from build123d import *

# Parameters (mm, degrees)
BOSS_EXTRUDE1_START            = -131.7625
BOSS_EXTRUDE1_DEPTH            = 60.325
F_5_0MM_DOWEL_HOLE1_AT_2_COUNT = 2
F_5_0MM_DOWEL_HOLE1_AT_2_PITCH = 12.7
F_5_0MM_DOWEL_HOLE1_AT_3_COUNT = 2
F_5_0MM_DOWEL_HOLE1_AT_3_PITCH = 28.398063314
F_5_0MM_DOWEL_HOLE1_AT_4_COUNT = 2
F_5_0MM_DOWEL_HOLE1_AT_4_PITCH = 25.4
F_5_0MM_DOWEL_HOLE1_AT_5_COUNT = 2
F_5_0MM_DOWEL_HOLE1_AT_5_PITCH = 50.8
F_5_0MM_DOWEL_HOLE1_AT_6_COUNT = 2
F_5_0MM_DOWEL_HOLE1_AT_6_PITCH = 52.363441445
FILLET2_R                      = 2.54
FILLET3_R                      = 2.54
FILLET4_R                      = 2.54
F_5_0MM_DOWEL_HOLE2_AT_2_COUNT = 2
F_5_0MM_DOWEL_HOLE2_AT_2_PITCH = 41.275
F_5_0MM_DOWEL_HOLE2_AT_3_COUNT = 2
F_5_0MM_DOWEL_HOLE2_AT_3_PITCH = 45.459081876
F_5_0MM_DOWEL_HOLE2_AT_4_COUNT = 2
F_5_0MM_DOWEL_HOLE2_AT_4_PITCH = 50.624060678
F_5_0MM_DOWEL_HOLE2_AT_5_COUNT = 2
F_5_0MM_DOWEL_HOLE2_AT_5_PITCH = 29.3116
F_5_0MM_DOWEL_HOLE2_AT_6_COUNT = 2
F_5_0MM_DOWEL_HOLE2_AT_6_PITCH = 19.05


with BuildPart() as part:
    # Sketch5 → Boss-Extrude1 (new body)
    with BuildSketch(Plane.XY.offset(BOSS_EXTRUDE1_START)):
        Polygon((50.8, 99.695), (50.8, 98.1075), (138.43, 98.1075), (215.9, 98.1075), (215.9, 99.695), align=None)
    extrude(amount=BOSS_EXTRUDE1_DEPTH)

    # Sketch7 → Ø5.0mm Dowel Hole1 (revolve, cut)
    with BuildSketch(Plane(origin=(114.3, 99.695, -107.95), x_dir=(0, 0, 1), z_dir=(1, 0, 0))):
        Polygon((0, 0), (0, 1.5875), (2.5, 1.5875), (2.5, 0.025), (2.525, 0), align=None)
    f_5_0mm_dowel_hole1 = revolve(axis=Axis((114.3, 106.045, -107.95), (0, -1, 0)), mode=Mode.SUBTRACT)

    # Ø5.0mm Dowel Hole1 at 2: Ø5.0mm Dowel Hole1 ×2
    with Locations(*[(0, 0, i * F_5_0MM_DOWEL_HOLE1_AT_2_PITCH) for i in range(1, F_5_0MM_DOWEL_HOLE1_AT_2_COUNT)]):
        add(f_5_0mm_dowel_hole1, mode=Mode.SUBTRACT)

    # Ø5.0mm Dowel Hole1 at 3: Ø5.0mm Dowel Hole1 ×2
    with Locations(*[Vector(-0.894427190999915, 0, 0.44721359549996) * (i * F_5_0MM_DOWEL_HOLE1_AT_3_PITCH) for i in range(1, F_5_0MM_DOWEL_HOLE1_AT_3_COUNT)]):
        add(f_5_0mm_dowel_hole1, mode=Mode.SUBTRACT)

    # Ø5.0mm Dowel Hole1 at 4: Ø5.0mm Dowel Hole1 ×2
    with Locations(*[(-i * F_5_0MM_DOWEL_HOLE1_AT_4_PITCH, 0, 0) for i in range(1, F_5_0MM_DOWEL_HOLE1_AT_4_COUNT)]):
        add(f_5_0mm_dowel_hole1, mode=Mode.SUBTRACT)

    # Ø5.0mm Dowel Hole1 at 5: Ø5.0mm Dowel Hole1 ×2
    with Locations(*[(-i * F_5_0MM_DOWEL_HOLE1_AT_5_PITCH, 0, 0) for i in range(1, F_5_0MM_DOWEL_HOLE1_AT_5_COUNT)]):
        add(f_5_0mm_dowel_hole1, mode=Mode.SUBTRACT)

    # Ø5.0mm Dowel Hole1 at 6: Ø5.0mm Dowel Hole1 ×2
    with Locations(*[Vector(-0.9701425001453318, 0, 0.2425356250363337) * (i * F_5_0MM_DOWEL_HOLE1_AT_6_PITCH) for i in range(1, F_5_0MM_DOWEL_HOLE1_AT_6_COUNT)]):
        add(f_5_0mm_dowel_hole1, mode=Mode.SUBTRACT)

    # Fillet2
    # the kernel refuses this fillet: 2.54 mm, written as the material it takes off along each edge
    with BuildSketch(Plane(origin=(215.9, 99.695, -137.649107549), x_dir=(-1, 0, 0), z_dir=(0, 0, 1))) as fillet2_piece_1:
        with BuildLine():
            CenterArc((2.35464302, 2.54), FILLET2_R, 202.024312837, 67.975687163)
            Line((0, 1.5875), (-0.04709286, 1.56845))
            ThreePointArc((-0.04709286, 1.56845), (-0.0508, 0.79375), (-0.0508, 0))
            Line((-0.0508, 0), (0, -0.0508))
            Line((0, -0.0508), (2.35464302, -0.0508))
            Line((2.35464302, -0.0508), (2.35464302, 0))
        make_face()
    extrude(amount=72.098215098, mode=Mode.SUBTRACT)

    # Fillet3
    # the kernel refuses this fillet: 2.54 mm, written as the material it takes off along each edge
    with BuildSketch(Plane(origin=(221.786607549, 98.1075, -71.4375), x_dir=(0, 0, -1), z_dir=(-1, 0, 0))) as fillet3_piece_1:
        with BuildLine():
            CenterArc((2.35464302, -2.54), FILLET3_R, 90, 67.975687163)
            Line((0, -1.5875), (-0.04709286, -1.56845))
            ThreePointArc((-0.04709286, -1.56845), (-0.0508, -0.79375), (-0.0508, 0))
            Line((-0.0508, 0), (0, 0.0508))
            Line((0, 0.0508), (2.35464302, 0.0508))
            Line((2.35464302, 0.0508), (2.35464302, 0))
        make_face()
    extrude(amount=176.873215098, mode=Mode.SUBTRACT)

    # Fillet4
    # the kernel refuses this fillet: 2.54 mm, written as the material it takes off along each edge
    with BuildSketch(Plane(origin=(44.913392451, 98.1075, -131.7625), x_dir=(0, 1, 0), z_dir=(1, 0, 0))) as fillet4_piece_1:
        with BuildLine():
            CenterArc((2.54, 2.35464302), FILLET4_R, 180, 67.975687163)
            Line((0, 2.35464302), (-0.0508, 2.35464302))
            Line((-0.0508, 2.35464302), (-0.0508, 0))
            Line((-0.0508, 0), (0, -0.0508))
            ThreePointArc((0, -0.0508), (0.79375, -0.0508), (1.56845, -0.04709286))
            Line((1.56845, -0.04709286), (1.5875, 0))
        make_face()
    extrude(amount=176.873215098, mode=Mode.SUBTRACT)
    with BuildSketch(Plane(origin=(50.8, 98.1075, -137.649107549), x_dir=(0, 1, 0), z_dir=(0, 0, 1))) as fillet4_piece_2:
        with BuildLine():
            CenterArc((2.54, -2.35464302), FILLET4_R, 112.024312837, 67.975687163)
            Line((0, -2.35464302), (-0.0508, -2.35464302))
            Line((-0.0508, -2.35464302), (-0.0508, 0))
            Line((-0.0508, 0), (0, 0.0508))
            ThreePointArc((0, 0.0508), (0.79375, 0.0508), (1.56845, 0.04709286))
            Line((1.56845, 0.04709286), (1.5875, 0))
        make_face()
    extrude(amount=69.743572079, mode=Mode.SUBTRACT)

    # Sketch9 → Ø5.0mm Dowel Hole2 (revolve, cut)
    with BuildSketch(Plane(origin=(167.083317581, 99.695, -122.2375), x_dir=(0, 0, 1), z_dir=(1, 0, 0))):
        Polygon((0, 0), (0, 1.5875), (2.5, 1.5875), (2.5, 0.025), (2.525, 0), align=None)
    f_5_0mm_dowel_hole2 = revolve(axis=Axis((167.083317581, 106.045, -122.2375), (0, -1, 0)), mode=Mode.SUBTRACT)

    # Ø5.0mm Dowel Hole2 at 2: Ø5.0mm Dowel Hole2 ×2
    with Locations(*[(0, 0, i * F_5_0MM_DOWEL_HOLE2_AT_2_PITCH) for i in range(1, F_5_0MM_DOWEL_HOLE2_AT_2_COUNT)]):
        add(f_5_0mm_dowel_hole2, mode=Mode.SUBTRACT)

    # Ø5.0mm Dowel Hole2 at 3: Ø5.0mm Dowel Hole2 ×2
    with Locations(*[Vector(0.41905817746174606, 0, 0.9079593845004521) * (i * F_5_0MM_DOWEL_HOLE2_AT_3_PITCH) for i in range(1, F_5_0MM_DOWEL_HOLE2_AT_3_COUNT)]):
        add(f_5_0mm_dowel_hole2, mode=Mode.SUBTRACT)

    # Ø5.0mm Dowel Hole2 at 4: Ø5.0mm Dowel Hole2 ×2
    with Locations(*[Vector(0.5790053110568745, 0, 0.8153237699024432) * (i * F_5_0MM_DOWEL_HOLE2_AT_4_PITCH) for i in range(1, F_5_0MM_DOWEL_HOLE2_AT_4_COUNT)]):
        add(f_5_0mm_dowel_hole2, mode=Mode.SUBTRACT)

    # Ø5.0mm Dowel Hole2 at 5: Ø5.0mm Dowel Hole2 ×2
    with Locations(*[(i * F_5_0MM_DOWEL_HOLE2_AT_5_PITCH, 0, 0) for i in range(1, F_5_0MM_DOWEL_HOLE2_AT_5_COUNT)]):
        add(f_5_0mm_dowel_hole2, mode=Mode.SUBTRACT)

    # Ø5.0mm Dowel Hole2 at 6: Ø5.0mm Dowel Hole2 ×2
    with Locations(*[(i * F_5_0MM_DOWEL_HOLE2_AT_6_PITCH, 0, 0) for i in range(1, F_5_0MM_DOWEL_HOLE2_AT_6_COUNT)]):
        add(f_5_0mm_dowel_hole2, mode=Mode.SUBTRACT)


solid = part.part
Source: CAD feature listing. Evaluate the final solid. Frame: model axes, mm. Coordinates: 2 decimals unless noted, no trailing zeros.
Item 1: Material intervals for line 1 (Z direction, x = 114.3, y = 98.75); line 2 (X direction, y = 98.9, z = -95.25); line 3 (X direction, y = 99.2, z = -107.95), sorted ascending.
Output values:
line 1: z = -131.1 to -110.45, -105.45 to -97.75, -92.75 to -72.1
line 2: x = 51.31 to 61, 66 to 86.4, 91.4 to 111.8, 116.8 to 215.39
line 3: x = 51.07 to 61, 66 to 86.4, 91.4 to 111.8, 116.8 to 215.05
Item 2: Cut plane A-A (x = 88.9). Count the separate pieces of the cut face and the enclosed holes in it, plus the area to 3 significant figures.
Output values:
separate pieces: 3
enclosed holes: 0
area: 77.8 mm2
Item 3: Pull-direction query (X, two-part tool) for faces 1 (the face through (133, 98.108, -102)), 2 (the face through (62.749, 98.9, -105.565)), 3 (the face through (86.42, 98.9, -108.28)); classes: pulls with the +X half, pulls with the -X half, needs draft (parallel to the pull), parting line crosses it, or undercut.
Output values:
face 1: needs draft
face 2: undercut
face 3: undercut
Item 4: First-contact query: P1, Ø4, axis at x = 114.3, z = -95.25, coming from the +Y side. Flat tip, straight axial feed; report the tip coordinate or a pass-through.
Output values:
P1: passes through
